The figure shows three views and two pictorial views of one solid part (mm, origin at its lowest corner). Answer the questions. A direction names the side the tool comes from. Give positions to 0.01 mm unless a question says otherwise; leave off trailing zeros. Loops run counter-clockwise (first coordinate to the right, second up) from the corner with the lowest first, then second, coordinate; pieces in that order, holes last. Notation, with made-up numbers: (-6, -23) - (5, -23) arc R18 ccw to (5, 7) - close; hole circle Ø4 at (35, 64). An arc over 180 degrees is marked (long way). Write each question's results on one line, items separated by ' | '.
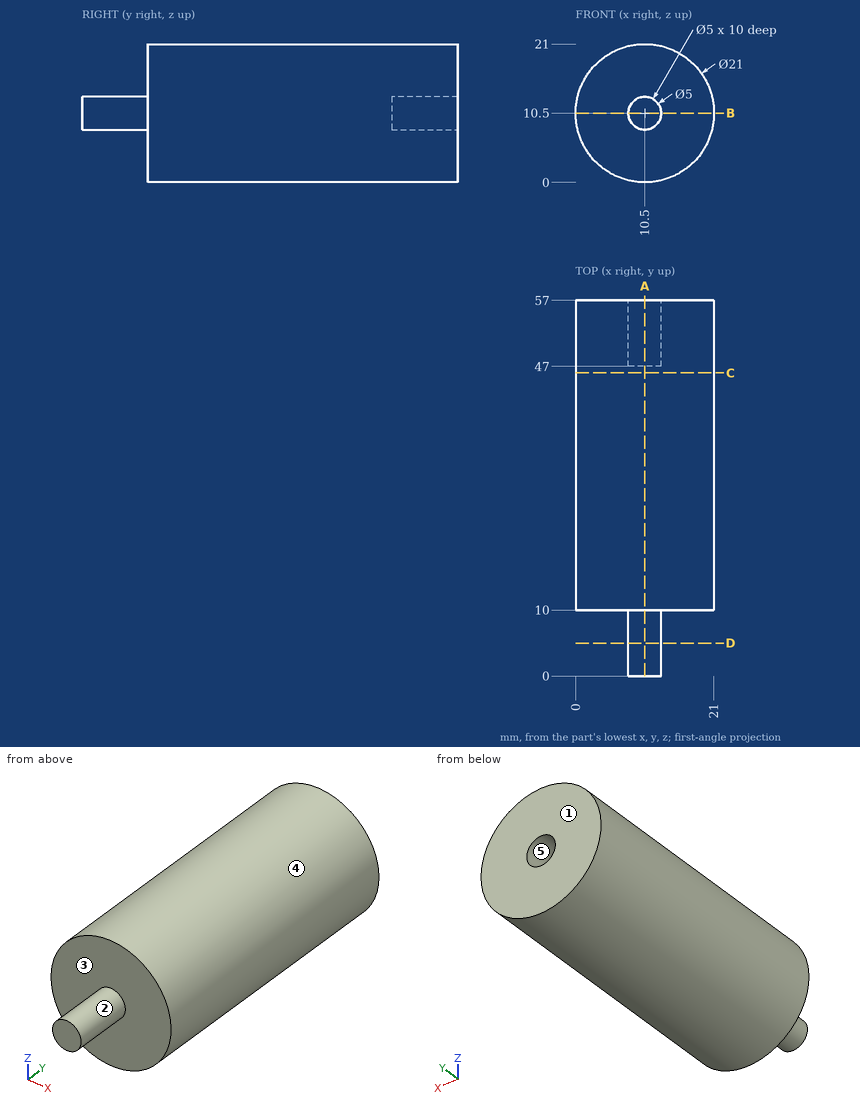
Item 1: For a pull along Z with two mould halves and no side action, classify the marked faces 3, 4 and 5 as released by +Z, released by -Z, zero draft, split by the parting line, or undercut.
Values found:
face 3: zero draft | face 4: split by the parting line | face 5: undercut
Item 2: A cutting plane is placed at C-C, the plane y = 46. Determine the outline of the cut face in (x, z).
Values found:
outline: circle Ø21 at (10.5, 10.5)
Item 3: Flat-ended cylindrical pins translate along their axes: P1, Ø12, axis at x = 18.5, y = 46.5, coming from the +Z side; P2, Ø1.5, axis at x = 13, y = 7.5, coming from the -Z side; P3, Ø10, axis at y = 49, z = 2.5, coming from the -X side. Find the tip coordinate at first contact, or state that the pin passes through.
Values found:
P1: stops at z = 20.81 | P2: stops at z = 8.71 | P3: stops at x = 0.44
Item 4: Find the intervals of material crossed by line 1 along X through (y, z) = (51.25, 10.5); line 2 along Y through (x, z) = (10.75, 17.25); line 3 along Y through (x, z) = (9, 10.75), in increasing order. Write a range as [from, to].
Values found:
line 1: x = [0, 8], [13, 21] | line 2: y = [10, 57] | line 3: y = [0, 47]
Item 5: For the marked faces 1 and 2, determine the directions among +Z, -Z, +X, -X, +Y, -Y from which every point of the face is accessible in a straight line to the end or side of a thin tool.
Values found:
face 1: +Z, -Z, +X, -X, +Y | face 2: -Y
Item 6: A cutting plane is placed at B-B, the plane z = 10.5. Determine the outline of the cut face in (x, y), plus the area to 3 significant figures.
Values found:
outline: (0, 10) - (8, 10) - (8, 0) - (13, 0) - (13, 10) - (21, 10) - (21, 57) - (13, 57) - (13, 47) - (8, 47) - (8, 57) - (0, 57) - close | area: 987 mm²
Item 7: A cutting plane is placed at A-A, the plane x = 10.5. Determine the outline of the cut face in (y, z).
Values found:
outline: (0, 8) - (10, 8) - (10, 0) - (57, 0) - (57, 8) - (47, 8) - (47, 13) - (57, 13) - (57, 21) - (10, 21) - (10, 13) - (0, 13) - close
Item 8: A cutting plane is placed at D-D, the plane y = 5. Determine the outline of the cut face in (x, z).
Values found:
outline: circle Ø5 at (10.5, 10.5)
